from build123d import *

# Parameters (mm, degrees)
SKETCH2_W            = 130
SKETCH2_H            = 130
BOSS_EXTRUDE1_DEPTH  = 100
SKETCH3_W            = 104
SKETCH3_H            = 74
CUT_EXTRUDE1_DEPTH   = 127
SKETCH4_W            = 10
SKETCH4_H            = 10
CUT_EXTRUDE3_DEPTH   = 105
SKETCH5_W            = 104
SKETCH5_H            = 10
CUT_EXTRUDE4_DEPTH   = 127
SKETCH6_W            = 10
SKETCH6_H            = 74
CUT_EXTRUDE5_DEPTH   = 127
SKETCH7_R            = 1.75
CUT_EXTRUDE6_DEPTH   = 20
SKETCH8_W            = 3
SKETCH8_H            = 3
CUT_EXTRUDE7_DEPTH   = 5
SKETCH9_W            = 85
SKETCH9_H            = 60
BOSS_EXTRUDE2_DEPTH  = 15
SKETCH11_W           = 85
SKETCH11_H           = 6
BOSS_EXTRUDE5_DEPTH  = 5
SKETCH12_W           = 85
SKETCH12_H           = 3
CUT_EXTRUDE9_DEPTH   = 4
SKETCH13_W           = 82
SKETCH13_H           = 57
CUT_EXTRUDE10_DEPTH  = 15
SKETCH15_W           = 3
SKETCH15_H           = 3
BOSS_EXTRUDE7_DEPTH  = 5
SKETCH16_W           = 82
SKETCH16_H           = 2
BOSS_EXTRUDE8_DEPTH  = 57
SKETCH17_W           = 77
SKETCH17_H           = 47
CUT_EXTRUDE11_DEPTH  = 10
SKETCH19_W           = 7
SKETCH19_H           = 2
SKETCH19_H_2         = 1
BOSS_EXTRUDE9_DEPTH  = 1
SKETCH21_W           = 3
SKETCH21_H           = 3
CUT_EXTRUDE15_DEPTH  = 5
SKETCH22_W           = 124
SKETCH22_H           = 7
BOSS_EXTRUDE10_DEPTH = 127
SKETCH23_W           = 120
SKETCH23_H           = 3
CUT_EXTRUDE16_DEPTH  = 125
SKETCH24_W           = 120
SKETCH24_H           = 110
CUT_EXTRUDE17_DEPTH  = 15
SKETCH25_W           = 71
SKETCH25_H           = 88
CUT_EXTRUDE18_DEPTH  = 15
SKETCH27_W           = 103
SKETCH27_H           = 17
BOSS_EXTRUDE11_DEPTH = 127
SKETCH28_W           = 97
SKETCH28_H           = 3
SKETCH28_H_2         = 10
CUT_EXTRUDE19_DEPTH  = 120
SKETCH29_W           = 4
SKETCH29_H           = 103
CUT_EXTRUDE20_DEPTH  = 17
SKETCH30_W           = 115
SKETCH30_H           = 87
CUT_EXTRUDE21_DEPTH  = 17


with BuildPart() as part:
    # Sketch2 → Boss-Extrude1 (new body)
    with BuildSketch(Plane(origin=(0, 0, 0), x_dir=(1, 0, 0), z_dir=(0, 1, 0))):
        with Locations((65, 65)):
            Rectangle(SKETCH2_W, SKETCH2_H)
    extrude(amount=BOSS_EXTRUDE1_DEPTH)

    # Sketch3 → Cut-Extrude1 (cut)
    with BuildSketch(Plane.ZY):
        with Locations((-65, 50)):
            Rectangle(SKETCH3_W, SKETCH3_H)
    extrude(amount=-CUT_EXTRUDE1_DEPTH, mode=Mode.SUBTRACT)

    # Sketch4 → Cut-Extrude3 (cut)
    with BuildSketch(Plane(origin=(130, 0, 0), x_dir=(0, 0, -1), z_dir=(1, 0, 0))):
        with Locations((5, 95)):
            Rectangle(SKETCH4_W, SKETCH4_H)
        with Locations((125, 95)):
            Rectangle(SKETCH4_W, SKETCH4_H)
        with Locations((5, 5)):
            Rectangle(SKETCH4_W, SKETCH4_H)
        with Locations((125, 5)):
            Rectangle(SKETCH4_W, SKETCH4_H)
    extrude(amount=-CUT_EXTRUDE3_DEPTH, mode=Mode.SUBTRACT)

    # Sketch5 → Cut-Extrude4 (cut)
    with BuildSketch(Plane.ZY):
        with Locations((-65, 92)):
            Rectangle(SKETCH5_W, SKETCH5_H)
        with Locations((-65, 8)):
            Rectangle(SKETCH5_W, SKETCH5_H)
    extrude(amount=-CUT_EXTRUDE4_DEPTH, mode=Mode.SUBTRACT)

    # Sketch6 → Cut-Extrude5 (cut)
    with BuildSketch(Plane.ZY):
        with Locations((-122, 50)):
            Rectangle(SKETCH6_W, SKETCH6_H)
        with Locations((-8, 50)):
            Rectangle(SKETCH6_W, SKETCH6_H)
    extrude(amount=-CUT_EXTRUDE5_DEPTH, mode=Mode.SUBTRACT)

    # Sketch7 → Cut-Extrude6 (cut)
    with BuildSketch(Plane.ZY):
        with Locations((-124, 94)):
            Circle(SKETCH7_R)
        with Locations((-6, 94)):
            Circle(SKETCH7_R)
        with Locations((-124, 6)):
            Circle(SKETCH7_R)
        with Locations((-6, 6)):
            Circle(SKETCH7_R)
    extrude(amount=-CUT_EXTRUDE6_DEPTH, mode=Mode.SUBTRACT)

    # Sketch8 → Cut-Extrude7 (cut)
    with BuildSketch(Plane.ZY):
        with Locations((-118.5, 88.5)):
            Rectangle(SKETCH8_W, SKETCH8_H)
        with Locations((-11.5, 88.5)):
            Rectangle(SKETCH8_W, SKETCH8_H)
        with Locations((-118.5, 11.5)):
            Rectangle(SKETCH8_W, SKETCH8_H)
        with Locations((-11.5, 11.5)):
            Rectangle(SKETCH8_W, SKETCH8_H)
    extrude(amount=-CUT_EXTRUDE7_DEPTH, mode=Mode.SUBTRACT)

    # Sketch9 → Boss-Extrude2 (add)
    with BuildSketch(Plane(origin=(0, 3, 0), x_dir=(1, 0, 0), z_dir=(0, 1, 0))):
        with Locations((42.5, 87)):
            Rectangle(SKETCH9_W, SKETCH9_H)
    extrude(amount=BOSS_EXTRUDE2_DEPTH)

    # Sketch11 → Boss-Extrude5 (add)
    with BuildSketch(Plane(origin=(0, 13, 0), x_dir=(1, 0, 0), z_dir=(0, 1, 0))):
        with Locations((42.5, 120)):
            Rectangle(SKETCH11_W, SKETCH11_H)
    extrude(amount=BOSS_EXTRUDE5_DEPTH)

    # Sketch12 → Cut-Extrude9 (cut)
    with BuildSketch(Plane(origin=(0, 18, 0), x_dir=(1, 0, 0), z_dir=(0, 1, 0))):
        with Locations((42.5, 121.5)):
            Rectangle(SKETCH12_W, SKETCH12_H)
    extrude(amount=-CUT_EXTRUDE9_DEPTH, mode=Mode.SUBTRACT)

    # Sketch13 → Cut-Extrude10 (cut)
    with BuildSketch(Plane(origin=(0, 18, 0), x_dir=(1, 0, 0), z_dir=(0, 1, 0))):
        with Locations((41, 88.5)):
            Rectangle(SKETCH13_W, SKETCH13_H)
    extrude(amount=-CUT_EXTRUDE10_DEPTH, mode=Mode.SUBTRACT)

    # Sketch15 → Boss-Extrude7 (add)
    with BuildSketch(Plane.ZY.offset(-5)):
        with Locations((-118.5, 11.5)):
            Rectangle(SKETCH15_W, SKETCH15_H)
    extrude(amount=BOSS_EXTRUDE7_DEPTH)

    # Sketch16 → Boss-Extrude8 (add)
    with BuildSketch(Plane(origin=(0, 0, -60), x_dir=(-1, 0, 0), z_dir=(0, 0, -1))):
        with Locations((-41, 17)):
            Rectangle(SKETCH16_W, SKETCH16_H)
        with Locations((-41, 12)):
            Rectangle(SKETCH16_W, SKETCH16_H)
    extrude(amount=BOSS_EXTRUDE8_DEPTH)

    # Sketch17 → Cut-Extrude11 (cut)
    with BuildSketch(Plane(origin=(0, 18, 0), x_dir=(1, 0, 0), z_dir=(0, 1, 0))):
        with Locations((38.5, 88.5)):
            Rectangle(SKETCH17_W, SKETCH17_H)
    extrude(amount=-CUT_EXTRUDE11_DEPTH, mode=Mode.SUBTRACT)

    # Sketch19 → Boss-Extrude9 (add)
    with BuildSketch(Plane.XY.offset(-117)):
        with Locations((3.5, 10)):
            Rectangle(SKETCH19_W, SKETCH19_H)
        with Locations((3.5, 13.5)):
            Rectangle(SKETCH19_W, SKETCH19_H_2)
    extrude(amount=BOSS_EXTRUDE9_DEPTH)

    # Sketch21 → Cut-Extrude15 (cut)
    with BuildSketch(Plane.ZY):
        with Locations((-118.5, 11.5)):
            Rectangle(SKETCH21_W, SKETCH21_H)
    extrude(amount=-CUT_EXTRUDE15_DEPTH, mode=Mode.SUBTRACT)

    # Sketch22 → Boss-Extrude10 (add)
    with BuildSketch(Plane.ZY.offset(-127)):
        with Locations((-65, 46.5)):
            Rectangle(SKETCH22_W, SKETCH22_H)
    extrude(amount=BOSS_EXTRUDE10_DEPTH)

    # Sketch23 → Cut-Extrude16 (cut)
    with BuildSketch(Plane.ZY):
        with Locations((-65, 46.5)):
            Rectangle(SKETCH23_W, SKETCH23_H)
    extrude(amount=-CUT_EXTRUDE16_DEPTH, mode=Mode.SUBTRACT)

    # Sketch24 → Cut-Extrude17 (cut)
    with BuildSketch(Plane(origin=(0, 50, 0), x_dir=(1, 0, 0), z_dir=(0, 1, 0))):
        with Locations((60, 65)):
            Rectangle(SKETCH24_W, SKETCH24_H)
    extrude(amount=-CUT_EXTRUDE17_DEPTH, mode=Mode.SUBTRACT)

    # Sketch25 → Cut-Extrude18 (cut)
    with BuildSketch(Plane(origin=(0, 100, 0), x_dir=(1, 0, 0), z_dir=(0, 1, 0))):
        with Locations((35.5, 65)):
            Rectangle(SKETCH25_W, SKETCH25_H)
    extrude(amount=-CUT_EXTRUDE18_DEPTH, mode=Mode.SUBTRACT)

    # Sketch27 → Boss-Extrude11 (add)
    with BuildSketch(Plane.ZY.offset(-127)):
        with Locations((-65, 88.5)):
            Rectangle(SKETCH27_W, SKETCH27_H)
    extrude(amount=BOSS_EXTRUDE11_DEPTH)

    # Sketch28 → Cut-Extrude19 (cut)
    with BuildSketch(Plane.ZY):
        with Locations((-65, 83.5)):
            Rectangle(SKETCH28_W, SKETCH28_H)
        with Locations((-65, 92)):
            Rectangle(SKETCH28_W, SKETCH28_H_2)
    extrude(amount=-CUT_EXTRUDE19_DEPTH, mode=Mode.SUBTRACT)

    # Sketch29 → Cut-Extrude20 (cut)
    with BuildSketch(Plane.XZ.offset(-80)):
        with Locations((125, -65)):
            Rectangle(SKETCH29_W, SKETCH29_H)
    extrude(amount=-CUT_EXTRUDE20_DEPTH, mode=Mode.SUBTRACT)

    # Sketch30 → Cut-Extrude21 (cut)
    with BuildSketch(Plane(origin=(0, 87, 0), x_dir=(1, 0, 0), z_dir=(0, 1, 0))):
        with Locations((57.5, 65)):
            Rectangle(SKETCH30_W, SKETCH30_H)
    extrude(amount=-CUT_EXTRUDE21_DEPTH, mode=Mode.SUBTRACT)


solid = part.part
Model file for the job. Use its own axes, mm. A direction names the side the tool comes from. Round coordinates to 2 decimals unless told otherwise and drop trailing zeros. Order: outer loops, then holes, each group sorted by start corner. A loop starts at its lowest first (then second) coordinate and runs counter-clockwise, first axis right, second up. Notation, with made-up numbers: M 43.25,68 L 57.25,68 A19 ccw 57.25,95 Z; hole C -17.5,64 d4. An arc over 180 degrees is marked long. Write each question's results on one line, items separated by ' | '. Start each with the question number.
(1) Probe probe 1 along Y at (x, z) = (34, -111.5); probe 2 along Y at (x, z) = (12.5, -122); probe 3 along Y at (x, z) = (12.25, -6). List the from-to ranges inside material, lowest first. Write a range as from..to.
(2) Saw through at A-A, the plane y = 94. Give the cut face in (x, z).
(3) Saw through at C-C, the plane x = 79. State how many separate pieces and enclosed holes the cut face has, then the cut area to 4 significant figures.
(4) Which spindle directions (+Z, -Z, +X, -X, +Y, -Y) get a long thin tool onto all of the face, cutting with end or side? Do faces 1 (the face through (78, 10, -125)), 2 (the face through (62, 88, -13.5)), 3 (the face through (78, 5, -10)), 4 (the face through (78, 95, -10)). Say none if no direction does.
(5) Two-plate mould, pull along X, no slides. Class faces 5 (the face through (117, 82, -65)), 6 (the face through (120, 92, -66)), 7 (the face through (127, 23, -66)): pulls with the +X half, pulls with the -X half, needs draft (parallel to the pull), parting line crosses it, or undercut.
(6) Saw through at D-D, the plane y = 68. Give the cut face in (x, z), then the cut area to 3 significant figures.
(7) Drop flat-ended pins along their axis: pin 1 (8.5 mm diameter, centred on x = 63.5, y = 84.5, fed in from +Z); pin 2 (0.6 mm diameter, centred on y = 81, z = -62.5, fed in from -X); pin 3 (1.5 mm diameter, centred on y = 12, z = -11, fed in from -X). Give the stop position or say it passes through.
(8) Saw through at B-B, the plane z = -44.5. Give the cut face in (x, y).
Established:
1) probe 1: y = 0..3, 80..82, 85..87, 97..100 | probe 2: y = 0..14, 43..45, 48..50, 87..100 | probe 3: y = 0..4.25, 7.75..13, 43..45, 48..50, 87..92.25, 95.75..100
2) outline: M 0,-130 L 25,-130 L 25,-120 L 130,-120 L 130,-10 L 25,-10 L 25,0 L 0,0 L 0,-4.25 L 20,-4.25 L 20,-7.75 L 0,-7.75 L 0,-13 L 127,-13 L 127,-117 L 0,-117 L 0,-122.25 L 20,-122.25 L 20,-125.75 L 0,-125.75 Z; M 0,-116.5 L 123,-116.5 L 123,-13.5 L 0,-13.5 L 0,-16.5 L 120,-16.5 L 120,-113.5 L 0,-113.5 Z
3) separate pieces: 1 | enclosed holes: 3 | area: 1,845 mm^2
4) face 1: -Z, +X, -Y | face 2: -X | face 3: +Z, +X, -Y | face 4: +Z, +X, +Y
5) face 5: needs draft | face 6: pulls with the -X half | face 7: undercut
6) outline: M 0,-130 L 130,-130 L 130,0 L 0,0 L 0,-3 L 127,-3 L 127,-127 L 0,-127 Z | area: 1,150 mm^2
7) pin 1: stops at z = 0 | pin 2: stops at x = 115 | pin 3: stops at x = 5
8) outline: M 0,0 L 130,0 L 130,100 L 71,100 L 71,97 L 120,97 L 120,87 L 115,87 L 115,85 L 120,85 L 120,82 L 115,82 L 115,80 L 123,80 L 123,97 L 127,97 L 127,50 L 120,50 L 120,48 L 125,48 L 125,45 L 120,45 L 120,43 L 127,43 L 127,3 L 0,3 Z
